from build123d import *

# Parameters (mm, degrees)
F0_W        = 69.85
F0_H        = 114.3
F0_R        = 3.81
F1_DEPTH    = 2.54
F2_T1_DEPTH = 89.4462243683
F2_T3_DEPTH = 133.8962243683


# Not quite as in the source:
# - a fillet or chamfer that OpenCascade refuses, or shapes differently, is made with other operations: its cross-section is extruded or revolved along the edge and cut away or added


with BuildPart() as f1:
    # F0 (on Front) → F1 (new body)
    with BuildSketch(Plane.XZ):
        with Locations((-0.3112182021, 0)):
            Rectangle(F0_W, F0_H)
        with Locations((0, -48.4124)):
            Circle(F0_R, mode=Mode.SUBTRACT)
        Polygon((-3.81, 11.43), (0, 11.43), (3.81, 11.43), (3.81, -11.43), (-3.81, -11.43), align=None, mode=Mode.SUBTRACT)
        with Locations((0, 48.4124)):
            Circle(F0_R, mode=Mode.SUBTRACT)
    extrude(amount=F1_DEPTH)

    # F2: chamfer of 3.81 on 4 edges, made by hand

    # F2_s2 → F2_t1 (cut)
    with BuildSketch(Plane.YZ.offset(-45.0343303863)):
        Polygon((-2.54, 53.34), (1.27, 57.15), (-2.54, 57.15), align=None)
        Polygon((-2.54, -53.34), (1.27, -57.15), (-2.54, -57.15), align=None)
    extrude(amount=F2_T1_DEPTH, mode=Mode.SUBTRACT)

    # F2_s4 → F2_t3 (cut)
    with BuildSketch(Plane.XY.offset(-66.9481121842)):
        Polygon((-31.4262182021, -2.54), (-35.2362182021, 1.27), (-35.2362182021, -2.54), align=None)
        Polygon((34.6137817979, 1.27), (30.8037817979, -2.54), (34.6137817979, -2.54), align=None)
    extrude(amount=F2_T3_DEPTH, mode=Mode.SUBTRACT)


solid = f1.part
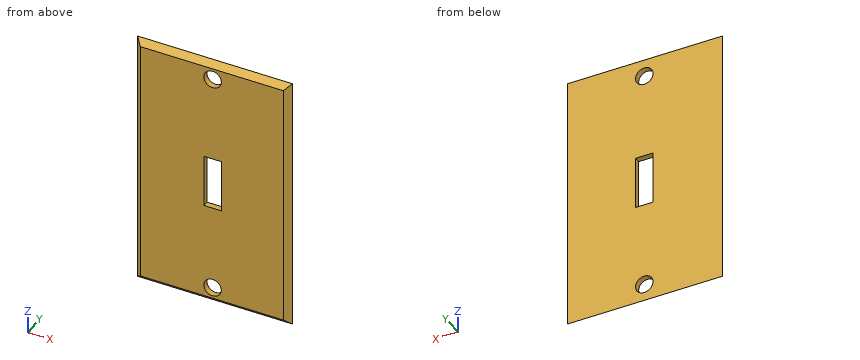
Input: part model. Units: mm. Frame: model coordinates. Coordinates: 2 decimals unless noted, no trailing zeros. Loops run counter-clockwise (first coordinate to the right, second up) from the corner with the lowest first, then second, coordinate; pieces in that order, holes last.
(1) Section A-A on x = 0. Return the cut outline in (y, z).
(2) First-contact query: pin 1 Ø9 at (x, z) = (0, -48.41) entering from +Y; pin 2 Ø1.3 at (x, y) = (0, -1) entering from +Z; pin 3 Ø1.5 at (x, y) = (-7.5, -2) entering from -Z; pin 4 Ø1.3 at (y, z) = (-1.5, -0.5) entering from -X. Flat tips, straight axial feed; report the tip coordinate or a pass-through.
(3) Section D-D on x = -8.5. Return the cut outline in (y, z).
(4) Material intervals for probe 1 along Z at (x, y) = (0.5, -1.95); probe 2 along Z at (x, y) = (-0.5, -2.15); probe 3 along X at (y, z) = (-0.1, 50.5), sorted ascending.
(5) Section B-B on y = -2.05. Return the cut outline in (x, z), then the cut area to 3 significant figures.
(6) Section C-C on z = 39. Return the cut outline in (x, y).
Data:
1. outline: (-2.54, -53.34) - (0, -55.88) - (0, -52.22) - (-2.54, -52.22) - close; (-2.54, -44.6) - (0, -44.6) - (0, -11.43) - (-2.54, -11.43) - close; (-2.54, 11.43) - (0, 11.43) - (0, 44.6) - (-2.54, 44.6) - close; (-2.54, 52.22) - (0, 52.22) - (0, 55.88) - (-2.54, 53.34) - close
2. pin 1: stops at y = 0
2. pin 2: stops at z = 55.53
2. pin 3: stops at z = -54.63
2. pin 4: stops at x = -33.12
3. outline: (-2.54, -53.34) - (0, -55.88) - (0, 55.88) - (-2.54, 53.34) - close
4. probe 1: z = -53.93 to -52.19, -44.64 to -11.43, 11.43 to 44.64, 52.19 to 53.93
4. probe 2: z = -53.73 to -52.19, -44.64 to -11.43, 11.43 to 44.64, 52.19 to 53.73
4. probe 3: x = -33.87 to -3.19, 3.19 to 33.24
5. outline: (-31.92, -53.83) - (31.29, -53.83) - (31.29, 53.83) - (-31.92, 53.83) - close; hole circle Ø7.62 at (0, -48.41); hole (-3.81, -11.43) - (3.81, -11.43) - (3.81, 11.43) - (-3.81, 11.43) - close; hole circle Ø7.62 at (0, 48.41)
5. area: 6,540 mm2
6. outline: (-33.97, 0) - (-31.43, -2.54) - (30.8, -2.54) - (33.34, 0) - close
